```python
from build123d import *

# Parameters (mm, degrees)
SKETCH001_W   = 81
SKETCH001_H   = 93
PAD_DEPTH     = 1.6
CHAMFER_SIZE  = 14
FILLET_R      = 4
SKETCH002_R   = 1.3
HOLE_DEPTH    = 1.601
SKETCH003_R   = 2
HOLE001_DEPTH = 1.601
SKETCH004_R   = 2
HOLE002_DEPTH = 1.601


with BuildPart() as part:
    # Sketch001 → Pad (new body)
    with BuildSketch(Plane.XY):
        Rectangle(SKETCH001_W, SKETCH001_H)
    extrude(amount=-PAD_DEPTH)

    # Chamfer
    chamfer_edges = [part.edges().sort_by_distance(p)[0] for p in [
        (-40.5, -46.5, -0.8),
        (40.5, -46.5, -0.8),
    ]]
    chamfer(chamfer_edges, length=CHAMFER_SIZE)

    # Fillet
    fillet_edges = [part.edges().sort_by_distance(p)[0] for p in [
        (-40.5, 46.5, -0.8),
        (40.5, 46.5, -0.8),
    ]]
    fillet(fillet_edges, radius=FILLET_R)

    # Sketch002 (on Face2 of Fillet) → Hole (cut, through all)
    with BuildSketch(Plane.XY):
        with Locations((-35.75, 41.8)):
            Circle(SKETCH002_R)
        with Locations((-35.75, 23.8)):
            Circle(SKETCH002_R)
        with Locations((35.75, 41.8)):
            Circle(SKETCH002_R)
        with Locations((35.75, 23.8)):
            Circle(SKETCH002_R)
        with Locations((-35.75, -10.8)):
            Circle(SKETCH002_R)
        with Locations((-35.75, -28.8)):
            Circle(SKETCH002_R)
        with Locations((35.75, -28.8)):
            Circle(SKETCH002_R)
        with Locations((35.75, -10.8)):
            Circle(SKETCH002_R)
    extrude(amount=-HOLE_DEPTH, mode=Mode.SUBTRACT)

    # Sketch003 (on Face2 of Hole) → Hole001 (cut, through all)
    with BuildSketch(Plane.XY):
        with Locations((-5.5, 41.5)):
            Circle(SKETCH003_R)
        with Locations((5.5, 41.5)):
            Circle(SKETCH003_R)
        with Locations((-29.428932, -36.5)):
            Circle(SKETCH003_R)
        with Locations((29.428932, -36.5)):
            Circle(SKETCH003_R)
    extrude(amount=-HOLE001_DEPTH, mode=Mode.SUBTRACT)

    # Sketch004 (on Face2 of Hole001) → Hole002 (cut, through all)
    with BuildSketch(Plane.XY):
        with Locations((-34.9, 6.5)):
            Circle(SKETCH004_R)
        with Locations((34.9, 6.5)):
            Circle(SKETCH004_R)
    extrude(amount=-HOLE002_DEPTH, mode=Mode.SUBTRACT)


solid = part.part
```
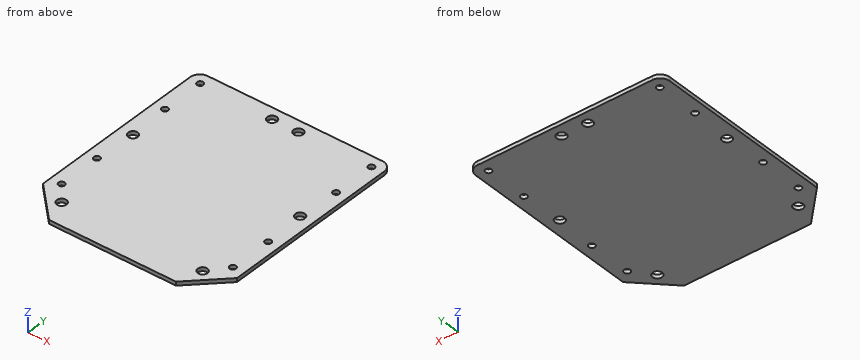
Geometry: final body of the model. Coordinates: model frame, mm. Coordinates: 2 decimals unless noted, no trailing zeros. Write each loop counter-clockwise with the first axis right and the second up, starting at its lowest first coordinate (ties: lowest second). Pieces come first, ordered by that corner, then holes. Notation, with made-up numbers: M 0.25,77 L 33.25,77 A27 ccw 33.25,102 Z; hole C 32,-2 d4. An arc over 180 degrees is marked long. Answer as CSV lines item,"result". Start each with the question number.
Q1. Cut plane A-A on x = -5.5. Return the cut outline in (y, z).
Q2. Cut plane D-D on y = -36.5. Return the cut outline in (x, z).
Q3. Cut plane B-B on y = 23.8. Return the cut outline in (x, z), then the cut area to 3 significant figures.
Q4. Cut plane C-C on z = -0.5. Count the separate pieces of the cut face and the enclosed holes in it, then the cut area to 3 significant figures.
Q5. Line query: line 1 (X direction, y = 41, z = -1.4); line 2 (Y direction, x = 35.75, z = -0.4). Output: solid intervals per line, ascending. Write a range as from..to.
Q6. Pin query (flat end, axial travel): P1, Ø6.5, axis at x = 34.9, y = 6.5, coming from the +Z side. Return the tip coordinate at first contact, or that it passes through.
Findings below:
1,outline,"M -46.5,-1.6 L 39.5,-1.6 L 39.5,0 L -46.5,0 Z; M 43.5,-1.6 L 46.5,-1.6 L 46.5,0 L 43.5,0 Z"
2,outline,"M -36.5,-1.6 L -31.43,-1.6 L -31.43,0 L -36.5,0 Z; M -27.43,-1.6 L 27.43,-1.6 L 27.43,0 L -27.43,0 Z; M 31.43,-1.6 L 36.5,-1.6 L 36.5,0 L 31.43,0 Z"
3,outline,"M -40.5,-1.6 L -37.05,-1.6 L -37.05,0 L -40.5,0 Z; M -34.45,-1.6 L 34.45,-1.6 L 34.45,0 L -34.45,0 Z; M 37.05,-1.6 L 40.5,-1.6 L 40.5,0 L 37.05,0 Z"
3,area,"121 mm2"
4,separate pieces,"1"
4,enclosed holes,"14"
4,area,"7,210 mm2"
5,line 1,"x = -40.5..-36.77, -34.73..-7.44, -3.56..3.56, 7.44..34.73, 36.77..40.5"
5,line 2,"y = -37.25..-30.1, -27.5..-12.1, -9.5..4.69, 8.31..22.5, 25.1..40.5, 43.1..46.5"
6,P1,"stops at z = 0"
